Here's how the part is built. I have some questions about the finished solid (model axes, mm). A direction names the side the tool comes from. Coordinates: 2 decimals unless noted, no trailing zeros. Write each loop counter-clockwise with the first axis right and the second up, starting at its lowest first coordinate (ties: lowest second). Pieces come first, ordered by that corner, then holes.
Item 1: I'm going to push flat-ended pins straight in: P1, Ø13.5, axis at x = 22.98, z = -31.81, coming from the +Y side; P2, Ø22, axis at x = -5.23, z = 11.53, coming from the +Y side. Where does each tip first touch, or does it pass through?
Item 2: I want a section at A-A (y = 7). Please give me the cut outline in (x, z) (3 decimals).
Item 3: If we mould it in two halves opening along X, with no side actions, what happens to faces 3 (the face through (50, 1, 1)), 4 (the face through (-1, -50, -1)), 5 (the face through (32, 46.42, 28))? For each: pulls with the +X half, pulls with the -X half, needs draft (parallel to the pull), parting line crosses it, or undercut.
Item 4: For faces 1 (the face through (-28, 46.42, 27)), 2 (the face through (-24.945, -1.115, -9.755)), which set-ups out of +Z, -Z, +X, -X, +Y, -Y let a thin tool reach every point of the face, with its end or its side?
Item 5: Please list where these lines run through material, in increasing order: line 1 (X direction, y = 4, z = 30); line 2 (Y direction, x = -26, z = -10); line 3 (X direction, y = -35, z = 28).
from build123d import *

# Parameters (mm, degrees)
SKETCH1_W                                       = 100
SKETCH1_H                                       = 100
BOSS_EXTRUDE1_DEPTH                             = 50
CSK_FOR_M2_FLAT_HEAD_MACHINE_SCREW1_D           = 17.07
CSK_FOR_M2_FLAT_HEAD_MACHINE_SCREW1_DEPTH       = 50.8
CSK_FOR_M2_FLAT_HEAD_MACHINE_SCREW1_CSINK_D     = 32.31
CSK_FOR_M2_FLAT_HEAD_MACHINE_SCREW1_CSINK_ANGLE = 100
CSK_FOR_M2_FLAT_HEAD_MACHINE_SCREW1_TIP         = 5.128345383
CBORE_FOR_M5_HEX_HEAD_BOLT1_AT_2_COUNT          = 2
CBORE_FOR_M5_HEX_HEAD_BOLT1_AT_2_PITCH          = 41.165028735
CBORE_FOR_M5_HEX_HEAD_BOLT1_AT_3_COUNT          = 2
CBORE_FOR_M5_HEX_HEAD_BOLT1_AT_3_PITCH          = 63.773894401


with BuildPart() as part:
    # Sketch1 → Boss-Extrude1 (new body, symmetric)
    with BuildSketch(Plane(origin=(0, 0, 0), x_dir=(1, 0, 0), z_dir=(0, 1, 0))):
        Rectangle(SKETCH1_W, SKETCH1_H)
    extrude(amount=BOSS_EXTRUDE1_DEPTH, both=True)

    # CSK for M2 Flat Head Machine Screw1
    with Locations(Plane(origin=(0, 50, 0), x_dir=(1, 0, 0), z_dir=(0, 1, 0))):
        with Locations((22.975631471, 31.812412806), (-5.231547771, -11.532234815)):
            CounterSinkHole(CSK_FOR_M2_FLAT_HEAD_MACHINE_SCREW1_D / 2, CSK_FOR_M2_FLAT_HEAD_MACHINE_SCREW1_CSINK_D / 2, depth=CSK_FOR_M2_FLAT_HEAD_MACHINE_SCREW1_DEPTH, counter_sink_angle=CSK_FOR_M2_FLAT_HEAD_MACHINE_SCREW1_CSINK_ANGLE)
            with Locations((0, 0, -(CSK_FOR_M2_FLAT_HEAD_MACHINE_SCREW1_DEPTH + CSK_FOR_M2_FLAT_HEAD_MACHINE_SCREW1_TIP / 2))):  # 118° drill point
                Cone(0, CSK_FOR_M2_FLAT_HEAD_MACHINE_SCREW1_D / 2, CSK_FOR_M2_FLAT_HEAD_MACHINE_SCREW1_TIP, mode=Mode.SUBTRACT)

    # Sketch10 → CBORE for M5 Hex Head Bolt1 (revolve, cut)
    with BuildSketch(Plane(origin=(-22.504336466, 50, -11.311080109), x_dir=(0, 0, 1), z_dir=(1, 0, 0))):
        Polygon((0, 0), (0, 100), (2.895, 100), (2.895, 3.58), (5.955, 3.58), (5.955, 0.532828266), (6.59, 0), align=None)
    cbore_for_m5_hex_head_bolt1 = revolve(axis=Axis((-22.504336466, 56.35, -11.311080109), (0, -1, 0)), mode=Mode.SUBTRACT)

    # CBORE for M5 Hex Head Bolt1 at 2: CBORE for M5 Hex Head Bolt1 ×2
    with Locations(*[Vector(-0.088729108, 0, 0.996055794) * (i * CBORE_FOR_M5_HEX_HEAD_BOLT1_AT_2_PITCH) for i in range(1, CBORE_FOR_M5_HEX_HEAD_BOLT1_AT_2_COUNT)]):
        add(cbore_for_m5_hex_head_bolt1, mode=Mode.SUBTRACT)

    # CBORE for M5 Hex Head Bolt1 at 3: CBORE for M5 Hex Head Bolt1 ×2
    with Locations(*[Vector(0.809215173, 0, 0.587512386) * (i * CBORE_FOR_M5_HEX_HEAD_BOLT1_AT_3_PITCH) for i in range(1, CBORE_FOR_M5_HEX_HEAD_BOLT1_AT_3_COUNT)]):
        add(cbore_for_m5_hex_head_bolt1, mode=Mode.SUBTRACT)


solid = part.part
Answer:
1. P1: stops at y = -1.87
1. P2: stops at y = 45.68
2. outline: (-50, -50) - (50, -50) - (50, 50) - (-50, 50) - close; hole circle Ø5.79 at (-26.157, 29.692); hole circle Ø5.79 at (-22.504, -11.311); hole circle Ø17.07 at (-5.232, 11.532); hole circle Ø17.07 at (22.976, -31.812); hole circle Ø5.79 at (29.102, 26.157)
3. face 3: pulls with the +X half
3. face 4: needs draft
3. face 5: undercut
4. face 1: +Y
4. face 2: +Y, -Y
5. line 1: x = -50 to -29.04, -23.28 to 50
5. line 2: y = -50 to 46.42
5. line 3: x = -50 to -28.51, -23.81 to 26.87, 31.33 to 50
